CAD build for the part. Positions are in the model's coordinates, mm. Face numbers are marked on the shaded views. A direction names the side the tool comes from. Round coordinates to 2 decimals unless told otherwise and drop trailing zeros. Loops run counter-clockwise (first coordinate to the right, second up) from the corner with the lowest first, then second, coordinate; pieces in that order, holes last. Notation, with made-up numbers: (23, -15.5) - (37, -15.5) arc R20 ccw to (37, -1.5) - close; hole circle Ø3 at (34, 21). An arc over 180 degrees is marked (long way). One line per question, with ' | ' between items.
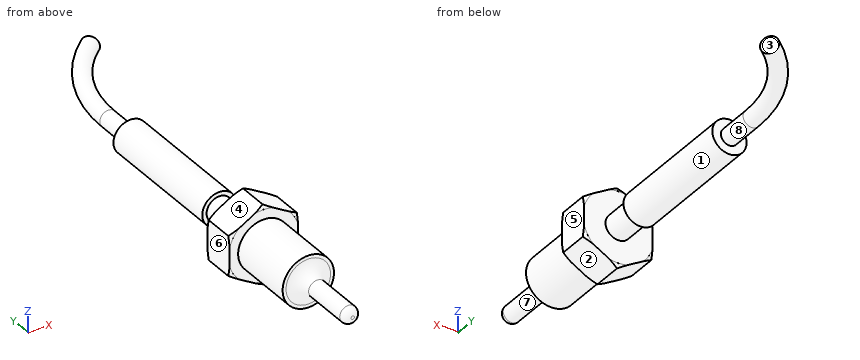
```python
from build123d import *

# Parameters (mm, degrees)
SKETCH2_OUTSIDE_W  = 41.992
SKETCH2_OUTSIDE_H  = 41.992
CUT_EXTRUDE1_DEPTH = 64.5
FILLET1_R          = 2.54
FILLET2_R          = 1.27
SWEEP1_PROFILE_R   = 1.5875


with BuildPart() as part:
    # Sketch1 → Revolve1 (revolve)
    with BuildSketch(Plane.XY):
        Polygon((0, 0), (0, 63.5), (3.175, 63.5), (3.175, 38.1), (2.38125, 38.1), (2.38125, 31.75), (12.7, 31.75), (12.7, 25.4), (4.7625, 25.4), (4.7625, 12.7), (1.5875, 12.7), (1.5875, 0), align=None)
    revolve(axis=Axis((0, 0, 0), (0, -1, 0)))

    # Sketch2 outside → Cut-Extrude1 (cut, through all)
    with BuildSketch(Plane(origin=(0, 0, 0), x_dir=(1, 0, 0), z_dir=(0, 1, 0))):
        Rectangle(SKETCH2_OUTSIDE_W, SKETCH2_OUTSIDE_H)
        Polygon((6.35, 3.666174209), (0, 7.332348419), (-6.35, 3.666174209), (-6.35, -3.666174209), (0, -7.332348419), (6.35, -3.666174209), align=None, mode=Mode.SUBTRACT)
    extrude(amount=CUT_EXTRUDE1_DEPTH, mode=Mode.SUBTRACT)

    # Sketch3 → Cut-Revolve1 (revolve, cut)
    with BuildSketch(Plane(origin=(0, 0, 0), x_dir=(0, 0, -1), z_dir=(1, 0, 0))):
        with BuildLine():
            Line((7.332348419, 31.369), (7.332348419, 25.781))
            ThreePointArc((7.332348419, 25.781), (6.9545441, 25.584108638), (6.570348419, 25.4))
            ThreePointArc((6.570348419, 25.4), (12.560590782, 25.250588883), (17.545931088, 28.575))
            ThreePointArc((17.545931088, 28.575), (12.560590782, 31.899411117), (6.570348419, 31.75))
            ThreePointArc((6.570348419, 31.75), (6.9545441, 31.565891362), (7.332348419, 31.369))
        make_face()
    revolve(axis=Axis((0, 0, 0), (0, 1, 0)), mode=Mode.SUBTRACT)

    # Fillet1
    fillet1_edges = [part.edges().sort_by_distance(p)[0] for p in [
        (-1.5875, 12.7, 0),
    ]]
    fillet(fillet1_edges, radius=FILLET1_R)

    # Fillet2
    fillet2_edges = [part.edges().sort_by_distance(p)[0] for p in [
        (-1.5875, 0, 0),
    ]]
    fillet(fillet2_edges, radius=FILLET2_R)

    # Sweep1: sweep along a path in Sketch4
    with BuildLine(Plane.XY) as sweep1_path:
        Line((0, 63.5), (0, 69.85))
        ThreePointArc((0, 69.85), (2.504749401, 80.848522628), (9.525, 89.677868645))
    # Sweep1 profile (on start of the path) → Sweep1 (sweep)
    with BuildSketch(Plane.ZX.offset(63.5)):
        Circle(SWEEP1_PROFILE_R)
    sweep(path=sweep1_path.line)


solid = part.part
```
(1) Drop flat-ended pins along their axis: P1, Ø3, axis at x = -4, z = 2.5, coming from the +Y side; P2, Ø1.5, axis at x = 2.5, y = 35.5, coming from the +Z side; P3, Ø5, axis at x = 7.5, z = -1, coming from the -Y side. Give the stop position or say it passes through.
Results found:
P1: stops at y = 31.75 | P2: stops at z = 1.61 | P3: stops at y = 25.4
(2) Two-plate mould, pull along Y, no slides. Class the marked faces 1, 2 and 3: released by +Y, released by -Y, zero draft, split by the parting line, or undercut.
Results found:
face 1: undercut | face 2: zero draft | face 3: released by +Y
(3) Tool access for the marked faces 4, 5, 6, 7 and 8: list every direction of +Z, -Z, +X, -X, +Y, -Y with a clear straight run to the whole face (end or side of a thin tool).
Results found:
face 4: +Z, -X, +Y, -Y | face 5: +Z, -Z, +X, -Y | face 6: +Z, -Z, -X, +Y, -Y | face 7: -Y | face 8: none
(4) Cut at B-B, the plane y = 35. Write the cut outline in (x, z).
Results found:
outline: circle Ø4.76 at (0, 0)
(5) Cut at A-A, the plane y = 47. Write the cut outline in (x, z) (3 decimals).
Results found:
outline: circle Ø6.35 at (0, 0)
(6) Probe L1, parallel to X at y = 29.5, z = 1.25; L2, parallel to Y at x = 0.5, z = -5.5; L3, parallel to Y at x = 2.75, z = -2.5. List the from-to ranges inside material, lowest first.
Results found:
L1: x = -6.35 to 6.35 | L2: y = 25.4 to 31.75 | L3: y = 12.67 to 31.75
